Work out the finished part from the listing and answer in its coordinate system (mm). A direction names the side the tool comes from. Give positions to 0.01 mm unless a question says otherwise; leave off trailing zeros. Loops run counter-clockwise (first coordinate to the right, second up) from the corner with the lowest first, then second, coordinate; pieces in that order, holes last. Notation, with made-up numbers: (46.5, -37.5) -> (64.5, -37.5) arc R18 ccw to (64.5, -22.5) -> close; hole circle Ø6 at (37, -24.75). An arc over 180 degrees is marked (long way). Answer as CSV lines item,"result". Start each with the question number.
1. Flat-ended cylindrical pins translate along their axes: pin 1 Ø8 at (y, z) = (-14.5, 7) entering from -X; pin 2 Ø1 at (y, z) = (11, 14) entering from +X; pin 3 Ø1.5 at (x, y) = (-8, 18.5) entering from +Z. Find the tip coordinate at first contact, or state that the pin passes through.
2. Determine the mould class of faces 1 (the face through (-5.799, -26.114, 10.628)), 2 (the face through (-14, 22, 20)), 3 (the face through (-3.22, 24.54, 10.88)) for opening direction Y: +Y half, -Y half, draft (parallel to the pull), parting line (faces both ways), or undercut.
3. Find the intervals of material crossed by line 1 along Y through (x, z) = (0, 12.25); line 2 along Z through (x, y) = (14, 7); line 3 along Y through (x, z) = (-5.5, 13.75), in increasing order.
4. Find section C-C, the plane z = 17.25. Give the vertices of the cut face in (x, y), and give its area (3 significant figures).
5. A tool of negligible diameter and unlimited length cuts with its end or side. For faces 4 (the face through (19.03, -19.03, 2)), 5 (the face through (-6.341, -28.554, 0.993)), from which of +Z, -Z, +X, -X, +Y, -Y can it reach the whole face along a straight path? Write none if from no direction.
6. Find section A-A, the plane x = 0. Give the vertices of the cut face in (y, z).
from build123d import *

# Parameters (mm, degrees)
SKETCH2_R           = 26.75
SKETCH2_R_2         = 29.25
SKETCH2_R_3         = 24.75
BOSS_EXTRUDE1_DEPTH = 2
SKETCH2_3_R         = 26.75
SKETCH2_3_R_2       = 24.75
BOSS_EXTRUDE2_DEPTH = 20
CHAMFER1_SIZE       = 0.5


with BuildPart() as part:
    # Sketch2 → Boss-Extrude1 (new body)
    with BuildSketch(Plane.XY):
        Circle(SKETCH2_R)
        Circle(SKETCH2_R_2)
        Circle(SKETCH2_R, mode=Mode.SUBTRACT)
        Circle(SKETCH2_R_3)
    extrude(amount=BOSS_EXTRUDE1_DEPTH)

    # Sketch2<3> → Boss-Extrude2 (add)
    with BuildSketch(Plane.XY):
        Circle(SKETCH2_3_R)
        Circle(SKETCH2_3_R_2, mode=Mode.SUBTRACT)
    extrude(amount=BOSS_EXTRUDE2_DEPTH)

    # Chamfer1
    chamfer1_edges = [part.edges().sort_by_distance(p)[0] for p in [
        (-26.75, 0, 20),
        (-29.25, 0, 0),
        (-29.25, 0, 2),
        (-24.75, 0, 2),
        (-24.75, 0, 20),
    ]]
    chamfer(chamfer1_edges, length=CHAMFER1_SIZE)


solid = part.part
Resolved:
1,pin 1,"stops at x = -24.6"
1,pin 2,"stops at x = 24.6"
1,pin 3,"stops at z = 2"
2,face 1,"parting line"
2,face 2,"draft"
2,face 3,"undercut"
3,line 1,"y = -26.75 to -24.75, 24.75 to 26.75"
3,line 2,"z = 0 to 2"
3,line 3,"y = -26.18 to -24.13, 24.13 to 26.18"
4,outline,"circle Ø53.5 at (0, 0); hole circle Ø49.5 at (0, 0)"
4,area,"324 mm^2"
5,face 4,"+Z"
5,face 5,"+Z, -Z"
6,outline,"(-29.25, 0.5) -> (-28.75, 0) -> (28.75, 0) -> (29.25, 0.5) -> (29.25, 1.5) -> (28.75, 2) -> (26.75, 2) -> (26.75, 19.5) -> (26.25, 20) -> (25.25, 20) -> (24.75, 19.5) -> (24.75, 2.5) -> (24.25, 2) -> (-24.25, 2) -> (-24.75, 2.5) -> (-24.75, 19.5) -> (-25.25, 20) -> (-26.25, 20) -> (-26.75, 19.5) -> (-26.75, 2) -> (-28.75, 2) -> (-29.25, 1.5) -> close"
